Geometry: final body of the model. Coordinates: model frame, mm. Face numbers are marked on the shaded views. Round coordinates to 2 decimals unless told otherwise and drop trailing zeros. Loops run counter-clockwise (first coordinate to the right, second up) from the corner with the lowest first, then second, coordinate; pieces in that order, holes last. Notation, with made-up numbers: M 36.5,-12.5 L 93.5,-12.5 A22 cw 93.5,-4.5 Z; hole C -13,64 d7. An arc over 180 degrees is marked long. Answer as a JSON object with one key per item and string values.
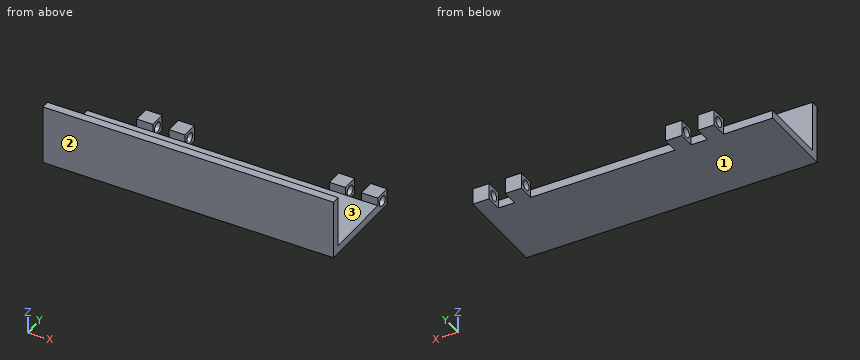
```python
from build123d import *

# Parameters (mm, degrees)
F0_W     = 28.575
F0_H     = 7.62
F1_DEPTH = 0.79375
F2_W     = 28.575
F2_H     = 0.79375
F3_DEPTH = 4.998339
F4_W     = 1.5875
F4_H     = 0.79375
F5_DEPTH = 1.5875
F6_W     = 1.5875
F6_H     = 1.5875
F7_DEPTH = 0.79375
F8_R     = 0.5
F9_DEPTH = 25.4


with BuildPart() as f1:
    # F0 (on Top) → F1 (new body)
    with BuildSketch(Plane.XY):
        with Locations((4.937336, 8.494605)):
            Rectangle(F0_W, F0_H)
    extrude(amount=F1_DEPTH)

    # F2 (on face) → F3 (join)
    with BuildSketch(Plane.XY.offset(0.79375)):
        with Locations((4.937336, 5.08148)):
            Rectangle(F2_W, F2_H)
    extrude(amount=F3_DEPTH)

    # F4 (on face) → F5 (join)
    with BuildSketch(Plane(origin=(0, 12.304605, 0), x_dir=(-1, 0, 0), z_dir=(0, 1, 0))):
        with Locations((-18.431086, 0.396875)):
            Rectangle(F4_W, F4_H)
        with Locations((-15.256086, 0.396875)):
            Rectangle(F4_W, F4_H)
        with Locations((0.523664, 0.396875)):
            Rectangle(F4_W, F4_H)
        with Locations((3.698664, 0.396875)):
            Rectangle(F4_W, F4_H)
    extrude(amount=F5_DEPTH)

    # F6 (on face) → F7 (join)
    with BuildSketch(Plane.XY.offset(0.79375)):
        with Locations((-3.698664, 13.098355)):
            Rectangle(F6_W, F6_H)
        with Locations((-0.523664, 13.098355)):
            Rectangle(F6_W, F6_H)
        with Locations((15.256086, 13.098355)):
            Rectangle(F6_W, F6_H)
        with Locations((18.431086, 13.098355)):
            Rectangle(F6_W, F6_H)
    extrude(amount=F7_DEPTH)

    # F8 (on face) → F9 (cut)
    with BuildSketch(Plane.YZ.offset(19.224836)):
        with Locations((13.098355, 0.79375)):
            Circle(F8_R)
    extrude(amount=-F9_DEPTH, mode=Mode.SUBTRACT)


solid = f1.part
```
1) Cut plane C-C on x = -5.25. Return the cut outline in (y, z), and give its area (3 significant figures).
Geometry results:
{"outline": "M 4.68,0 L 12.3,0 L 12.3,0.79 L 5.48,0.79 L 5.48,5.79 L 4.68,5.79 Z", "area": "10.0 mm2"}
2) Cut plane A-A on x = 15.5. Return the cut outline in (y, z).
Geometry results:
{"outline": "M 4.68,0 L 13.89,0 L 13.89,1.59 L 12.3,1.59 L 12.3,0.79 L 5.48,0.79 L 5.48,5.79 L 4.68,5.79 Z; hole C 13.1,0.79 d1"}
3) Pull-direction query (Y, two-part tool) for the marked faces 1, 2 and 3; classes: +Y half, -Y half, draft (parallel to the pull), parting line (faces both ways), or undercut.
Geometry results:
{"face 1": "draft", "face 2": "-Y half", "face 3": "undercut"}
4) Cut plane B-B on y = 13.25. Count the separate pieces of the cut face and the enclosed holes in it, and give its area (3 significant figures).
Geometry results:
{"separate pieces": "8", "enclosed holes": "0", "area": "4.03 mm2"}
5) Cut plane D-D on y = 6. Return the cut outline in (x, z), and give its area (3 significant figures).
Geometry results:
{"outline": "M -9.35,0 L 19.22,0 L 19.22,0.79 L -9.35,0.79 Z", "area": "22.7 mm2"}
6) First-contact query: pin 1 (1.3 mm diameter, centred on x = 18.5, y = 13.5, fed in from +Z); pin 2 (0.5 mm diameter, centred on y = 13, z = 0.5, fed in from -X); pin 3 (1.5 mm diameter, centred on x = 10, z = 3.5, fed in from +Y). Flat tips, straight axial feed; report the tip coordinate or a pass-through.
Geometry results:
{"pin 1": "z = 1.59", "pin 2": "x = -4.49", "pin 3": "y = 5.48"}
7) Line query: probe 1 along X at (y, z) = (12.5, 1.4); probe 2 along Z at (x, y) = (2.75, 12); probe 3 along Y at (x, z) = (6.75, 0.5). Output: solid intervals per line, ascending.
Geometry results:
{"probe 1": "-4.49 to -2.9, -1.32 to 0.27, 14.46 to 16.05, 17.64 to 19.22", "probe 2": "0 to 0.79", "probe 3": "4.68 to 12.3"}
